```python
from build123d import *

# Parameters (mm, degrees)
SKETCH1_R           = 1.65
SKETCH1_R_2         = 1.6
SKETCH1_R_3         = 2.65
BOSS_EXTRUDE1_DEPTH = 6


with BuildPart() as part:
    # Sketch1 → Boss-Extrude1 (new body)
    with BuildSketch(Plane(origin=(0, 6, 0), x_dir=(1, 0, 0), z_dir=(0, 1, 0))):
        with BuildLine():
            Line((104, 0), (55, 0))
            ThreePointArc((55, 0), (53.585786438, -0.585786438), (53, -2))
            Line((53, -2), (53, -18))
            ThreePointArc((53, -18), (53.585786438, -19.414213562), (55, -20))
            Line((55, -20), (71, -20))
            ThreePointArc((71, -20), (72.414213562, -20.585786438), (73, -22))
            Line((73, -22), (73, -43))
            ThreePointArc((73, -43), (73.585786438, -44.414213562), (75, -45))
            Line((75, -45), (91, -45))
            ThreePointArc((91, -45), (92.414213562, -44.414213562), (93, -43))
            Line((93, -43), (93, -36.5))
            ThreePointArc((93, -36.5), (95.928932188, -29.428932188), (103, -26.5))
            Line((103, -26.5), (104, -26.5))
            ThreePointArc((104, -26.5), (105.414213562, -25.914213562), (106, -24.5))
            Line((106, -24.5), (106, -2))
            ThreePointArc((106, -2), (105.414213562, -0.585786438), (104, 0))
        make_face()
        with Locations((99.5, -20)):
            Circle(SKETCH1_R, mode=Mode.SUBTRACT)
        with Locations((99.5, -7)):
            Circle(SKETCH1_R_2, mode=Mode.SUBTRACT)
        with Locations((83, -20)):
            Circle(SKETCH1_R_2, mode=Mode.SUBTRACT)
        with Locations((83, -10)):
            Circle(SKETCH1_R_3, mode=Mode.SUBTRACT)
        with Locations((60.5, -10)):
            Circle(SKETCH1_R_3, mode=Mode.SUBTRACT)
        with Locations((83, -37.5)):
            Circle(SKETCH1_R_3, mode=Mode.SUBTRACT)
    extrude(amount=-BOSS_EXTRUDE1_DEPTH)


solid = part.part
```
CAD build for the part. Positions are in the model's coordinates, mm. A direction names the side the tool comes from. Coordinates: 2 decimals unless noted, no trailing zeros. Loops run counter-clockwise (first coordinate to the right, second up) from the corner with the lowest first, then second, coordinate; pieces in that order, holes last. Notation, with made-up numbers: (47, -28) - (94, -28) arc R7 ccw to (94, -18) - close; hole circle Ø11 at (-28, 33.25). An arc over 180 degrees is marked (long way). Return JSON: item names as keys, results as strings.
1. 3-axis set-ups, long thin cutter, end or side, ignore diameter. For faces 4 (the cylindrical face through (62.95, 3.04, 11.01)), 5 (the flat face through (93, 3, 40)), 6 (the flat face through (63, 3, 20)): which of +Z, -Z, +X, -X, +Y, -Y reach the whole face in a straight line?
Result:
{"face 4": "+Y, -Y", "face 5": "+Z, +X, +Y, -Y", "face 6": "+Z, -X, +Y, -Y"}
2. Probe L1, parallel to Z at x = 83, y = 3.75; L2, parallel to Z at x = 60.5, y = 2.55; L3, parallel to Z at x = 99.5, y = 1.55. List the from-to ranges inside material, lowest first. Write a range as from..to.
Result:
{"L1": "z = 0..7.35, 12.65..18.4, 21.6..34.85, 40.15..45", "L2": "z = 0..7.35, 12.65..20", "L3": "z = 0..5.4, 8.6..18.35, 21.65..27.13"}
3. Band-saw the part on B-B (z = 10). Give the cut face in (x, y), and give its area (3 significant figures).
Result:
{"outline": "(53, 0) - (57.85, 0) - (57.85, 6) - (53, 6) - close; (63.15, 0) - (80.35, 0) - (80.35, 6) - (63.15, 6) - close; (85.65, 0) - (106, 0) - (106, 6) - (85.65, 6) - close", "area": "254 mm2"}
4. Band-saw the part on C-C (x = 83). Give the cut face in (y, z), and give its area (3 significant figures).
Result:
{"outline": "(0, 0) - (6, 0) - (6, 7.35) - (0, 7.35) - close; (0, 12.65) - (6, 12.65) - (6, 18.4) - (0, 18.4) - close; (0, 21.6) - (6, 21.6) - (6, 34.85) - (0, 34.85) - close; (0, 40.15) - (6, 40.15) - (6, 45) - (0, 45) - close", "area": "187 mm2"}
5. Mould opens along Z. For faces 1 (the cylindrical face through (82.792, 3.042, 18.414)), 2 (the flat face through (53, 3, 10)), 3 (the cylindrical face through (95.85, 3.04, 29.51)) say: released by +Z, released by -Z, zero draft, split by the parting line, or undercut.
Result:
{"face 1": "undercut", "face 2": "zero draft", "face 3": "released by +Z"}
6. Band-saw the part on A-A (y = 4.3). Give the cut face in (x, z), and give its area (3 significant figures).
Result:
{"outline": "(53, 2) arc R2 ccw to (55, 0) - (104, 0) arc R2 ccw to (106, 2) - (106, 24.5) arc R2 ccw to (104, 26.5) - (103, 26.5) arc R10 cw to (93, 36.5) - (93, 43) arc R2 ccw to (91, 45) - (75, 45) arc R2 ccw to (73, 43) - (73, 22) arc R2 cw to (71, 20) - (55, 20) arc R2 ccw to (53, 18) - close; hole circle Ø5.3 at (60.5, 10); hole circle Ø5.3 at (83, 10); hole circle Ø5.3 at (83, 37.5); hole circle Ø3.2 at (83, 20); hole circle Ø3.3 at (99.5, 20); hole circle Ø3.2 at (99.5, 7)", "area": "1,570 mm2"}
7. Band-saw the part on D-D (x = 100.5). Give the cut face in (y, z).
Result:
{"outline": "(0, 0) - (6, 0) - (6, 5.75) - (0, 5.75) - close; (0, 8.25) - (6, 8.25) - (6, 18.69) - (0, 18.69) - close; (0, 21.31) - (6, 21.31) - (6, 26.82) - (0, 26.82) - close"}
8. Drop flat-ended pins along their axis: pin 1 (3 mm diameter, centred on y = 4, z = 29, fed in from -X); pin 2 (0.5 mm diameter, centred on x = 103.5, y = 1.5, fed in from +Z); pin 3 (3 mm diameter, centred on y = 2, z = 39.5, fed in from +X). Give the stop position or say it passes through.
Result:
{"pin 1": "stops at x = 73", "pin 2": "stops at z = 26.5", "pin 3": "stops at x = 93"}
